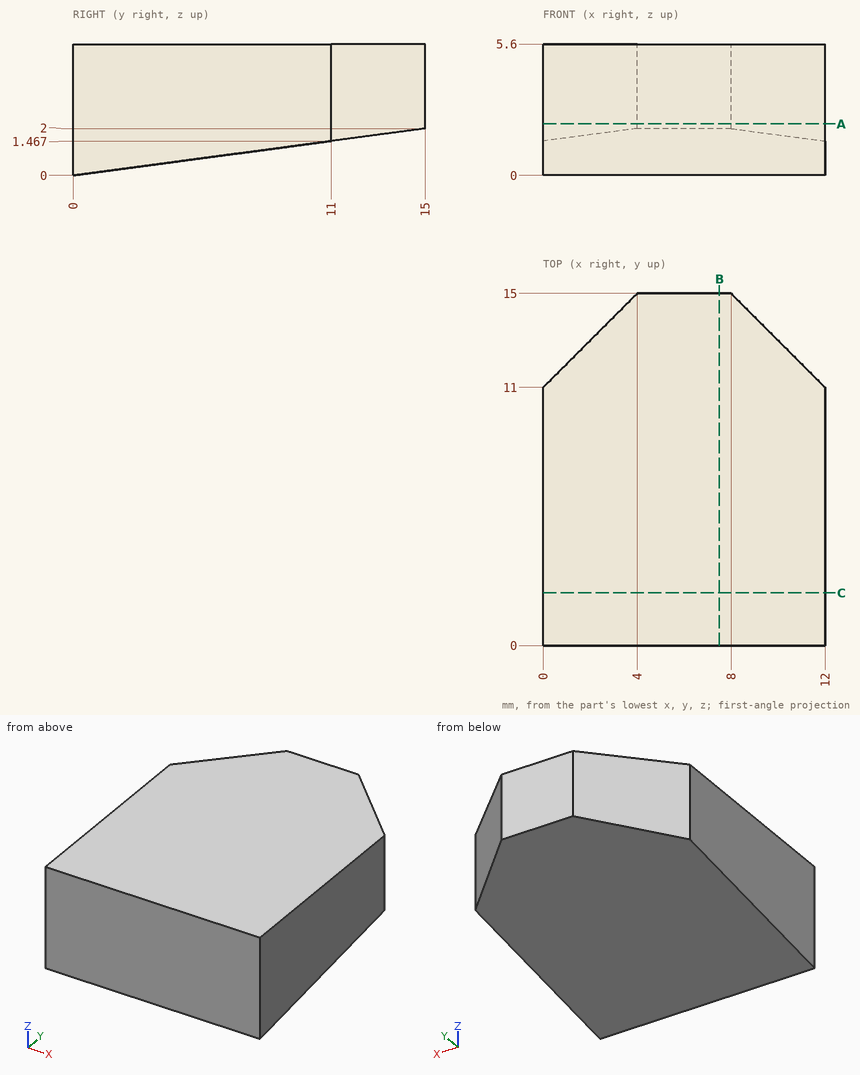
Geometry: see drawing. Coordinates: mm, zero at the bounding-box minimum. Round coordinates to 2 decimals unless told otherwise and drop trailing zeros. Write each loop counter-clockwise with the first axis right and the second up, starting at its lowest first coordinate (ties: lowest second). Pieces come first, ordered by that corner, then holes.
1) Contact query for flat-ended pins moving along their axis: P1, Ø3, axis at y = 13, z = 1.5, coming from the -X side; P2, Ø5, axis at x = 1.5, y = 12.5, coming from the -Z side; P3, Ø1.5, axis at x = 2, y = 10, coming from the -Z side. Output: stop coordinate, or through.
2) Cut plane C-C (y = 2.25). Return the cut outline in (x, z), then the cut area to 3 significant figures.
3) Ray query, L1, parallel to Y at x = 11, z = 3.35; L2, parallel to Z at x = 5, y = 14; L3, parallel to Y at x = 9.5, z = 2.4. Return the intervals inside material, ascending.
4) Cut plane B-B (x = 7.5). Return the cut outline in (y, z).
5) Cut plane A-A (z = 2.2). Return the cut outline in (x, y).
Geometry says:
1. P1: stops at x = 0.5
1. P2: stops at z = 1.33
1. P3: stops at z = 1.23
2. outline: (0, 0.3) - (12, 0.3) - (12, 5.6) - (0, 5.6) - close
2. area: 63.6 mm2
3. L1: y = 0 to 12
3. L2: z = 1.87 to 5.6
3. L3: y = 0 to 13.5
4. outline: (0, 0) - (15, 2) - (15, 5.6) - (0, 5.6) - close
5. outline: (0, 0) - (12, 0) - (12, 11) - (8, 15) - (4, 15) - (0, 11) - close
